Could you check a few things on this model? Use its own coordinates, in mm. Face numbers are marked on the shaded views. A direction names the side the tool comes from. Coordinates: 2 decimals unless noted, no trailing zeros. Order: outer loops, then holes, each group sorted by start corner. A loop starts at its lowest first (then second) coordinate and runs counter-clockwise, first axis right, second up. Notation, with made-up numbers: (36, 53.25) -> (87, 53.25) arc R30 ccw to (87, 87.25) -> close; hole circle Ø1 at (33.25, 33). An arc over 180 degrees is marked (long way). Use a Markdown table: item, result. Add a question column.
1) Thinking about a two-plate mould opening in Z: for the marked faces 4, 5 and 6, which applies, +Z half, -Z half, draft (parallel to the pull), parting line (faces both ways), or undercut?
2) If we section it at C-C (x = -3): Write out the boundary of the cut face in (y, z) (3 decimals), plus the area to 3 significant figures.
3) If we section it at B-B (y = 13): Write out the boundary of the cut face in (x, z) (3 decimals), plus the area to 3 significant figures.
4) Which directions (+Z, -Z, +X, -X, +Y, -Y) give clear straight access to the entire face, cutting with the end or side of a thin tool? Please do the marked faces 1, 2 and 3.
5) If we section it at D-D (z = -39.5): Write out the boundary of the cut face in (x, y) (3 decimals), plus the area to 3 significant figures.
6) If we section it at A-A (z = 5): Write out the boundary of the cut face in (x, y) (3 decimals).
7) If I drill on L1, parallel to Z at x = 3.5, y = 2; L2, parallel to Z at x = 5, y = 28; L3, parallel to X at y = 4, z = 49.5 (3 decimals), over which ranges is the centre line in solid material (lowest first)? Write a range as [from, to].
8) Will these pins go through, and if not, where does the flat tip stop? pin 1 Ø8 at (y, z) = (-0.5, 37.5) entering from +X; pin 2 Ø4 at (x, y) = (-1.5, 24) entering from +Z (3 decimals); pin 3 Ø5 at (x, z) = (-0.265, -56.81) entering from +Y; pin 4 Ø2.5 at (x, z) = (-0.5, 27.5) entering from +Y.
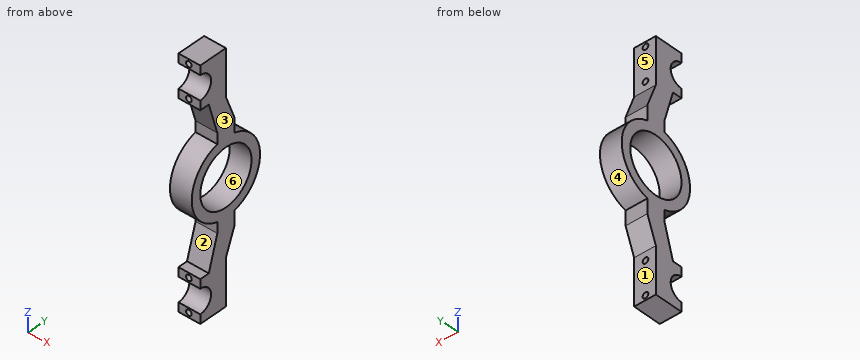
```python
from build123d import *

# Parameters (mm, degrees)
SKETCH1_R            = 5.765
SKETCH1_R_2          = 4.765
BOSS_EXTRUDE1_DEPTH  = 10
SKETCH2_W            = 11.53
SKETCH2_H            = 10
BOSS_EXTRUDE2_DEPTH  = 10
SKETCH3_R            = 4.765
CUT_EXTRUDE1_DEPTH   = 10
SKETCH8_W            = 11.53
SKETCH8_H            = 10
BOSS_EXTRUDE5_DEPTH  = 10
SKETCH9_R            = 3.5
CUT_EXTRUDE4_DEPTH   = 26.158316716
SKETCH11_W           = 11.53
SKETCH11_H           = 10
BOSS_EXTRUDE6_DEPTH  = 48.155
SKETCH12_R           = 6.35
BOSS_EXTRUDE7_DEPTH  = 5.765
SKETCH13_W           = 10
SKETCH13_H           = 20
CUT_EXTRUDE5_DEPTH   = 11.53
CUT_EXTRUDE6_DEPTH   = 11.53
MIRROR1_START        = -5.765
MIRROR1_DEPTH        = 11.53
MIRROR1_2_OUTLINE_R  = 6.35
MIRROR1_2_DEPTH      = 11.53
SKETCH15_W           = 10
SKETCH15_H           = 10
CUT_EXTRUDE7_DEPTH   = 11.53
SKETCH17_W           = 11.204655182
SKETCH17_H           = 10
BOSS_EXTRUDE10_DEPTH = 11.53
CUT_EXTRUDE9_DEPTH   = 74.053521476
SKETCH20_R           = 1.5
CUT_EXTRUDE10_DEPTH  = 73.36788877
SKETCH22_W           = 24.31
SKETCH22_H           = 5
CUT_EXTRUDE11_DEPTH  = 74.053521476
BOSS_EXTRUDE11_DEPTH = 11.53
SKETCH25_R           = 20
SKETCH25_R_2         = 15
BOSS_EXTRUDE12_DEPTH = 11.53
SKETCH26_R           = 15
CUT_EXTRUDE12_DEPTH  = 79.49724199


# Read off the part's stored shape, not the designer's step: Mirror1
with BuildPart() as part:
    # Sketch1 → Boss-Extrude1 (new body)
    with BuildSketch(Plane.XY):
        Circle(SKETCH1_R)
        Circle(SKETCH1_R_2, mode=Mode.SUBTRACT)
    extrude(amount=BOSS_EXTRUDE1_DEPTH)

    # Sketch2 → Boss-Extrude2 (add)
    with BuildSketch(Plane(origin=(0, 0, 0), x_dir=(1, 0, 0), z_dir=(0, 1, 0))):
        with Locations((0, -5)):
            Rectangle(SKETCH2_W, SKETCH2_H)
    extrude(amount=BOSS_EXTRUDE2_DEPTH)

    # Sketch3 → Cut-Extrude1 (cut)
    with BuildSketch(Plane(origin=(0, 0, 0), x_dir=(-1, 0, 0), z_dir=(0, 0, -1))):
        with Locations(Location((0, 0, 0), (0, 0, 180))):
            Circle(SKETCH3_R)
    extrude(amount=-CUT_EXTRUDE1_DEPTH, mode=Mode.SUBTRACT)

    # Sketch8 → Boss-Extrude5 (add)
    with BuildSketch(Plane(origin=(0, 10, 0), x_dir=(1, 0, 0), z_dir=(0, 1, 0))):
        with Locations((0, -5)):
            Rectangle(SKETCH8_W, SKETCH8_H)
    extrude(amount=BOSS_EXTRUDE5_DEPTH)

    # Sketch9 → Cut-Extrude4 (cut, through all)
    with BuildSketch(Plane(origin=(5.765, 0, 0), x_dir=(0, 0, -1), z_dir=(1, 0, 0))):
        with Locations((-5, 15)):
            Circle(SKETCH9_R)
    extrude(amount=-CUT_EXTRUDE4_DEPTH, mode=Mode.SUBTRACT)

    # Sketch11 → Boss-Extrude6 (add)
    with BuildSketch(Plane(origin=(0, 0, 0), x_dir=(-1, 0, 0), z_dir=(0, 0, -1))):
        with Locations((0, 15)):
            Rectangle(SKETCH11_W, SKETCH11_H)
    extrude(amount=BOSS_EXTRUDE6_DEPTH)

    # Sketch12 → Boss-Extrude7 (add, symmetric)
    with BuildSketch(Plane(origin=(0, 0, 0), x_dir=(0, 0, -1), z_dir=(1, 0, 0))):
        with BuildLine():
            Line((59.31, 0), (59.31, 20))
            Line((59.31, 20), (47, 20))
            Line((47, 20), (37, 20))
            Line((37, 20), (37, 0))
            ThreePointArc((37, 0), (48.155, -11.155), (59.31, 0))
        make_face()
        with Locations((48.155, 0)):
            Circle(SKETCH12_R, mode=Mode.SUBTRACT)
    extrude(amount=BOSS_EXTRUDE7_DEPTH, both=True)

    # Sketch13 → Cut-Extrude5 (cut)
    with BuildSketch(Plane.ZY.offset(5.765)):
        with Locations((5, 0)):
            Rectangle(SKETCH13_W, SKETCH13_H)
    extrude(amount=-CUT_EXTRUDE5_DEPTH, mode=Mode.SUBTRACT)

    # Sketch14 → Cut-Extrude6 (cut)
    with BuildSketch(Plane.ZY.offset(5.765)):
        Polygon((5, 18.5), (5, 10), (10, 10), (10, 18.5), (10, 20), (5, 20), align=None)
    extrude(amount=-CUT_EXTRUDE6_DEPTH, mode=Mode.SUBTRACT)

    # Mirror1 outline → Mirror1 (cut)
    with BuildSketch(Plane.YZ.offset(MIRROR1_START)):
        with BuildLine():
            Line((10, 5), (10, 0))
            Line((10, 0), (20, 0))
            Line((20, 0), (20, 5))
            Line((20, 5), (18.5, 5))
            ThreePointArc((18.5, 5), (15, 1.5), (11.5, 5))
            Line((11.5, 5), (10, 5))
        make_face()
    extrude(amount=MIRROR1_DEPTH, mode=Mode.SUBTRACT)

    # Mirror1 2 outline → Mirror1 2 (add)
    with BuildSketch(Plane.YZ.offset(MIRROR1_START)):
        with BuildLine():
            Line((0, 47), (10, 47))
            Line((10, 47), (10, 10))
            Line((10, 10), (0, 10))
            Line((0, 10), (0, 0))
            Line((0, 0), (10, 0))
            Line((10, 0), (10, 5))
            Line((10, 5), (11.5, 5))
            ThreePointArc((11.5, 5), (15, 8.5), (18.5, 5))
            Line((18.5, 5), (20, 5))
            Line((20, 5), (20, 69.31))
            Line((20, 69.31), (0, 69.31))
            ThreePointArc((0, 69.31), (-11.155, 58.155), (0, 47))
        make_face()
        with Locations((0, 58.155)):
            Circle(MIRROR1_2_OUTLINE_R, mode=Mode.SUBTRACT)
    extrude(amount=MIRROR1_2_DEPTH)

    # Sketch15 → Cut-Extrude7 (cut)
    with BuildSketch(Plane.ZY.offset(5.765)):
        with Locations((5, 5)):
            Rectangle(SKETCH15_W, SKETCH15_H)
    extrude(amount=-CUT_EXTRUDE7_DEPTH, mode=Mode.SUBTRACT)

    # Sketch17 → Boss-Extrude10 (add)
    with BuildSketch(Plane.ZY.offset(5.765)):
        with Locations((1.267367683, 15)):
            Rectangle(SKETCH17_W, SKETCH17_H)
    extrude(amount=-BOSS_EXTRUDE10_DEPTH)

    # Sketch19 → Cut-Extrude9 (cut, through all)
    with BuildSketch(Plane.ZY.offset(5.765)):
        Polygon((-41.805, 0), (69.31, 0), (69.31, -15), (-59.31, -15), (-59.31, 0), align=None)
    extrude(amount=-CUT_EXTRUDE9_DEPTH, mode=Mode.SUBTRACT)

    # Sketch20 → Cut-Extrude10 (cut, through all)
    with BuildSketch(Plane(origin=(0, 0, 0), x_dir=(-1, 0, 0), z_dir=(0, -1, 0))):
        with Locations(Location((0.265, 56.81, 0), (0, 0, 90))):
            Circle(SKETCH20_R)
        with Locations(Location((0.265, 39.5, 0), (0, 0, 90))):
            Circle(SKETCH20_R)
        with Locations(Location((0.265, -66.824084676, 0), (0, 0, 90))):
            Circle(SKETCH20_R)
        with Locations(Location((0.265, -49.5, 0), (0, 0, 90))):
            Circle(SKETCH20_R)
    extrude(amount=-CUT_EXTRUDE10_DEPTH, mode=Mode.SUBTRACT)

    # Sketch22 → Cut-Extrude11 (cut, through all)
    with BuildSketch(Plane(origin=(5.765, 0, 0), x_dir=(0, 0, -1), z_dir=(1, 0, 0))):
        Polygon((-32, 20), (-45, 20), (-45, 15), align=None)
        with Locations((-57.155, 17.5)):
            Rectangle(SKETCH22_W, SKETCH22_H)
        Polygon((35, 20), (22, 20), (35, 15), align=None)
        with Locations((47.155, 17.5)):
            Rectangle(SKETCH22_W, SKETCH22_H)
    extrude(amount=-CUT_EXTRUDE11_DEPTH, mode=Mode.SUBTRACT)

    # Sketch23 → Boss-Extrude11 (add)
    with BuildSketch(Plane(origin=(5.765, 0, 0), x_dir=(0, 0, -1), z_dir=(1, 0, 0))):
        Polygon((-47, 10), (-47, 5), (-30, 10), align=None)
        Polygon((37, 10), (20, 10), (37, 5), align=None)
    extrude(amount=-BOSS_EXTRUDE11_DEPTH)

    # Sketch25 → Boss-Extrude12 (add)
    with BuildSketch(Plane(origin=(5.765, 0, 0), x_dir=(0, 0, -1), z_dir=(1, 0, 0))):
        with Locations((-5, 15)):
            Circle(SKETCH25_R)
        with Locations((-5, 15)):
            Circle(SKETCH25_R_2, mode=Mode.SUBTRACT)
    extrude(amount=-BOSS_EXTRUDE12_DEPTH)

    # Sketch26 → Cut-Extrude12 (cut, through all)
    with BuildSketch(Plane(origin=(5.765, 0, 0), x_dir=(0, 0, -1), z_dir=(1, 0, 0))):
        with Locations((-5, 15)):
            Circle(SKETCH26_R)
    extrude(amount=-CUT_EXTRUDE12_DEPTH, mode=Mode.SUBTRACT)


solid = part.part
```
Answer sheet:
| question | item | result |
|---|---|---|
| 1 | face 4 | parting line |
| 1 | face 5 | draft |
| 1 | face 6 | undercut |
| 2 | outline | (0, -59.31) -> (15, -59.31) -> (15, -35) -> (20, -22) -> (20, -14.365) arc R20 ccw to (20, 24.365) -> (20, 32) -> (15, 45) -> (15, 69.31) -> (0, 69.31) -> (0, 64.505) arc R6.35 cw to (0, 51.805) -> (0, 47) -> (5, 47) -> (10, 30) -> (10, 24.365) arc R20 ccw to (10, -14.365) -> (10, -20) -> (5, -37) -> (0, -37) -> (0, -41.805) arc R6.35 cw to (0, -54.505) -> close; hole circle Ø30 at (15, 5) |
| 2 | area | 1,540 mm2 |
| 3 | outline | (-5.765, -59.31) -> (5.765, -59.31) -> (5.765, -9.866) -> (-5.765, -9.866) -> close; (-5.765, 19.866) -> (5.765, 19.866) -> (5.765, 69.31) -> (-5.765, 69.31) -> close; hole circle Ø3 at (-0.265, -56.81); hole circle Ø3 at (-0.265, -39.5); hole circle Ø3 at (-0.265, 49.5); hole circle Ø3 at (-0.265, 66.824) |
| 3 | area | 1,110 mm2 |
| 4 | face 1 | -Z, +X, -X, +Y |
| 4 | face 2 | +X, -X, -Y |
| 4 | face 3 | +Z, -Z, +X, +Y, -Y |
| 5 | outline | (-5.765, 0) -> (-1.765, 0) -> (-1.765, 15) -> (-5.765, 15) -> close; (1.235, 0) -> (5.765, 0) -> (5.765, 15) -> (1.235, 15) -> close |
| 5 | area | 128 mm2 |
| 6 | outline | (-5.765, -5) -> (5.765, -5) -> (5.765, 0) -> (-5.765, 0) -> close; (-5.765, 30) -> (5.765, 30) -> (5.765, 35) -> (-5.765, 35) -> close |
| 7 | L1 | [-59.31, -54.18], [-42.13, -37], [-10.2, -2.48], [12.48, 20.2], [47, 52.13], [64.18, 69.31] |
| 7 | L2 | [-10.2, -2.48], [12.48, 20.2] |
| 7 | L3 | [-5.765, -1.765], [1.235, 5.765] |
| 8 | pin 1 | through |
| 8 | pin 2 | z = 23.735 |
| 8 | pin 3 | y = 15 |
| 8 | pin 4 | y = 20 |
